Input: part model. Units: mm. Frame: model coordinates. Face numbers are marked on the shaded views. A direction names the side the tool comes from. Round coordinates to 2 decimals unless told otherwise and drop trailing zeros. Loops run counter-clockwise (first coordinate to the right, second up) from the corner with the lowest first, then second, coordinate; pieces in that order, holes last. Notation, with made-up numbers: (34, 72) -> (82, 72) arc R21 cw to (82, 99) -> close; hole circle Ø8 at (86.5, 77). An arc over 180 degrees is marked (long way). One line per question, with ' | ' between items. Start each with the question number.
Q1. Material intervals for L1, parallel to X at y = 0.75, z = -7.5; L2, parallel to Z at x = -12.75, y = -8.5, sorted ascending.
Q2. Cut plane B-B on x = -3.5. Return loops of the section in (y, z), and give its area (3 significant figures).
Q3. Cut plane C-C on z = -0.5. Return loops of the section in (x, y), and give its area (3 significant figures).
Q4. Access query for the marked faces 1, 2 and 3. Directions: +Z, -Z, +X, -X, +Y, -Y. A direction counts if a zero-diameter tool reaches every point of the face in a straight line with its end or side. Return the directions, or none.
Q5. Cut plane A-A on y = 1.75. Return loops of the section in (x, z), and give its area (3 significant figures).
Q6. Contact query for flat-ended pins moving along their axis: P1, Ø4.5, axis at x = -13, y = -6.5, coming from the +Z side; P2, Ø3, axis at x = -1, y = -8, coming from the +Z side; P3, Ø2, axis at x = -13, y = -6.5, coming from the -Z side; P4, Ø6, axis at y = -8, z = 0, coming from the -X side. Output: stop coordinate, or through.
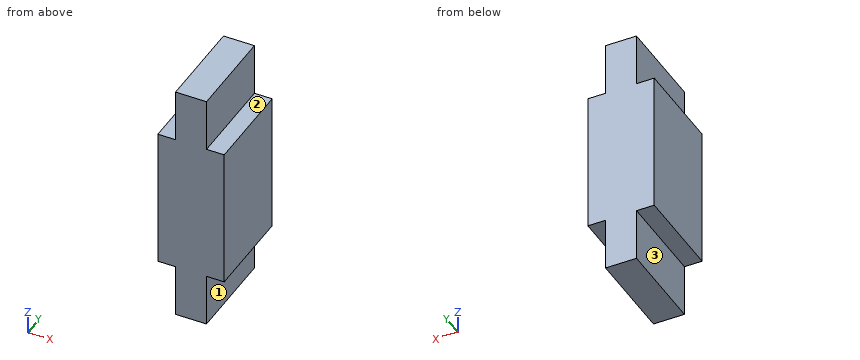
Autodesk Inventor part; units mm, degrees
ref_plane "YZ Plane" through (0, 0, 0) normal (1, 0, 0) x (0, 1, 0)
ref_plane "XZ Plane" through (0, 0, 0) normal (0, 1, 0) x (-1, 0, 0)
ref_plane "XY Plane" through (0, 0, 0) normal (0, 0, 1) x (1, 0, 0)
sketch "Sketch1" plane through (0, 0, 0) normal (0, 1, 0) x (-1, 0, 0)
  line L0 (4, 4) -> (11, 4)
  line L1 (11, -8) -> (4, -8)
  line L2 (11, -52) -> (4, -52)
  line L3 (4, -40) -> (11, -40)
  line L4 (15, -8) -> (0, -8)
  line L5 (0, -8) -> (0, -40)
  line L6 (0, -40) -> (15, -40)
  line L7 (15, -40) -> (15, -8)
  line L8 (11, 4) -> (11, -8)
  line L9 (4, 4) -> (4, -8)
  line L10 (4, -52) -> (4, -40)
  line L11 (11, -52) -> (11, -40)
  point P0 (4, 0)
  point P1 (11, 0)
  point P2 (11, -48)
  point P3 (4, -48)
  point P4 (0, -8)
  point P5 (15, -40)
extrude "Extrusion1" add sketch "Sketch1" against normal blind 15
sketch "Sketch2" plane through (0, 0, 0) normal (0, 1, 0) x (1, 0, 0)
  line L0 (-4, 8) -> (0, 8)
  line L1 (0, 8) -> (0, 40)
  line L2 (0, 40) -> (-4, 40)
  line L3 (-11, 40) -> (-15, 40)
  line L4 (-15, 40) -> (-15, 8)
  line L5 (-15, 8) -> (-11, 8)
  line L6 (-11, 52) -> (-4, 52)
  line L7 (-4, 40) -> (-11, 40)
  line L8 (-4, -4) -> (-11, -4)
  line L9 (-11, 8) -> (-4, 8)
  line L10 (-11, 52) -> (-11, 40)
  line L11 (-11, 8) -> (-11, -4)
  line L12 (-11, -4) -> (-4, -4)
  line L13 (-4, -4) -> (-4, 8)
  line L14 (-4, 40) -> (-4, 52)
  line L15 (-4, 52) -> (-11, 52)
  line L16 (-4, 52) -> (-4, 40)
  line L17 (-11, 52) -> (-11, 40)
  line L18 (-11, -4) -> (-11, 8)
  line L19 (-4, -4) -> (-4, 8)
  point P0 (-4, 0)
  point P1 (-4, 48)
  point P2 (-11, 48)
  point P3 (-11, 0)
extrude "Extrusion2" add sketch "Sketch2" along normal blind 6
sketch "Sketch3" plane through (0, 0, -52) normal (0, 0, -1) x (-1, 0, 0)
  line L0 (4, 6) -> (11, 6)
  line L1 (11, -15) -> (4, -15)
  line L2 (11, 6) -> (11, -15)
  line L3 (4, -15) -> (4, 6)
  point P0 (0, 0)
properties part number "Connector"
Results:
1) L1: -11 to -4 | L2: -40 to -8
2) outline: (-15, -40) -> (6, -40) -> (6, -8) -> (-15, -8) -> close | area: 672 mm^2
3) outline: (-11, -15) -> (-4, -15) -> (-4, 6) -> (-11, 6) -> close | area: 147 mm^2
4) face 1: -Z, +X, +Y, -Y | face 2: +Z, +X, +Y, -Y | face 3: -Z, -X, +Y, -Y
5) outline: (-15, -40) -> (-11, -40) -> (-11, -52) -> (-4, -52) -> (-4, -40) -> (0, -40) -> (0, -8) -> (-4, -8) -> (-4, 4) -> (-11, 4) -> (-11, -8) -> (-15, -8) -> close | area: 648 mm^2
6) P1: z = 4 | P2: z = -8 | P3: z = -40 | P4: x = -11
